The drawing under review shows one solid part. Ordinate dimensions are in mm from its lowest x, y, z. Coordinates: 2 decimals unless noted, no trailing zeros. Order: outer loops, then holes, each group sorted by start corner. A loop starts at its lowest first (then second) coordinate and runs counter-clockwise, first axis right, second up.
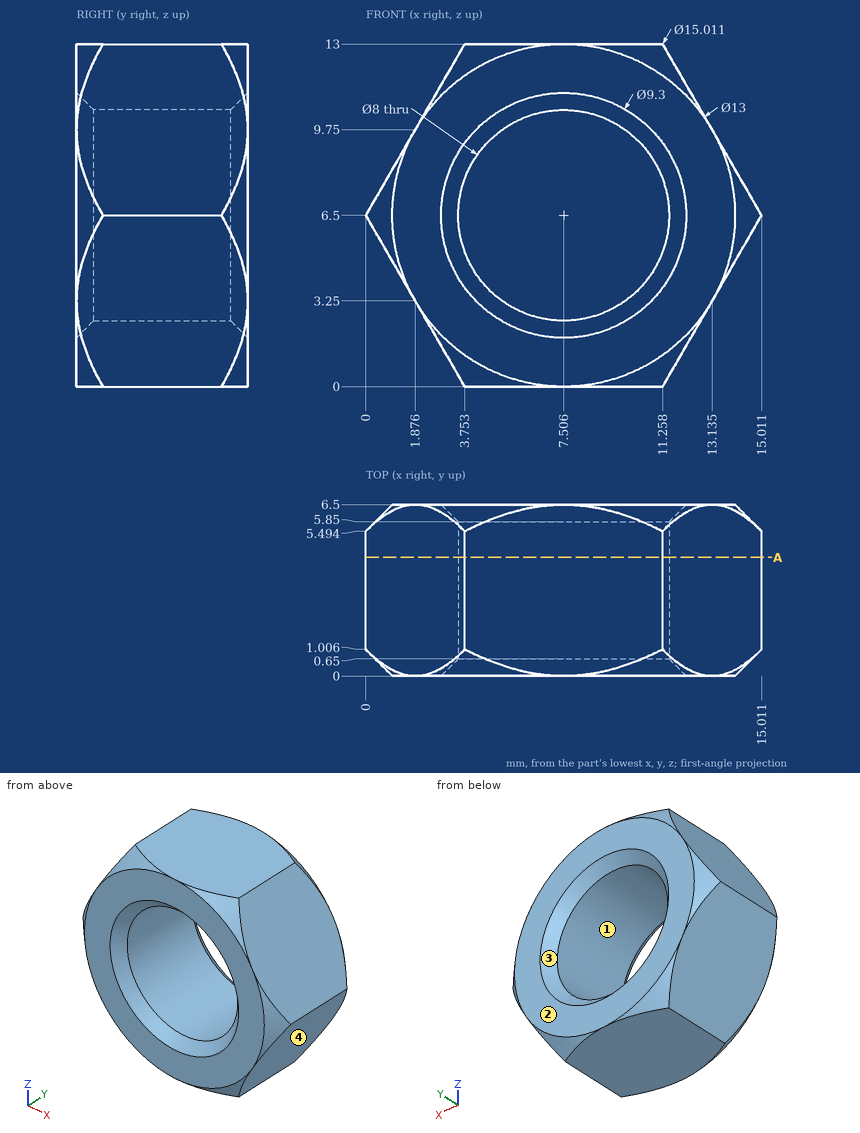
(1) Insertion check: pin 1 Ø1 at (x, y) = (4.5, 2.5) entering from -Z; pin 2 Ø3 at (y, z) = (2, 9) entering from +X (1 decimal); pin 3 Ø2 at (y, z) = (1.5, 10.5) entering from -X. Each pin has a flat end and moves straight along its axis. Give the tip position at first contact, or say it passes through.
(2) Consider section A-A (y = 4.5). Give the boundary of the cut face in (x, z) (1 decimal).
(3) The part is to be moulded in two halves that separate along X. For the marked faces 1, 2, 3 and 4, say which applies: +X half, -X half, draft (parallel to the pull), parting line (faces both ways), or undercut.
(4) Wall thickness on line 1 (Z direction, x = 6, y = 3.5) (1 decimal); line 2 (Z direction, x = 9.5, y = 2.5); line 3 (X direction, y = 1.75, z = 7.5) (1 decimal): over which ranges is each line inside the solid? List them lowest first.
Findings:
1. pin 1: stops at z = 0
1. pin 2: stops at x = 14.4
1. pin 3: stops at x = 1.73
2. outline: (0, 6.5) - (3.8, 0) - (11.3, 0) - (15, 6.5) - (11.3, 13) - (3.8, 13) - close; hole circle Ø8 at (7.5, 6.5)
3. face 1: undercut
3. face 2: draft
3. face 3: undercut
3. face 4: +X half
4. line 1: z = 0 to 2.8, 10.2 to 13
4. line 2: z = 0 to 3.03, 9.97 to 13
4. line 3: x = 0.6 to 3.6, 11.4 to 14.4
